CAD build for the part. Positions are in the model's coordinates, mm. Face numbers are marked on the shaded views. A direction names the side the tool comes from. Round coordinates to 2 decimals unless told otherwise and drop trailing zeros. Write each loop counter-clockwise with the first axis right and the second up, starting at its lowest first coordinate (ties: lowest second). Pieces come first, ordered by that corner, then holes. Notation, with made-up numbers: (-4.75, 9) -> (23.25, 9) arc R5 cw to (23.25, 17) -> close; hole circle Ø4 at (78, 28.5). An arc over 180 degrees is marked (long way). Put each result on its own line as item: value. Start each with the question number.
1. 3-axis set-ups, long thin cutter, end or side, ignore diameter. For the marked faces 1, 2 and 3: which of +Z, -Z, +X, -X, +Y, -Y reach the whole face in a straight line?
2. Drill centre lines: line 1 (X direction, y = 13, z = 1); line 2 (Z direction, x = 17, y = 2.5); line 3 (Z direction, x = 10.5, y = 27). Where is each one in solid material? Low to high. Write a range as from..to.
3. Saw through at A-A on y = 10. List the corners of the cut face in (x, z).
4. Saw through at D-D on x = 125. List the corners of the cut face in (y, z).
5. Saw through at C-C on z = 12.5. List the corners of the cut face in (x, y), and give its area (3 significant figures).
6. Flat gauge pins, fed straight in: P1, Ø10, axis at x = 80, z = 8, coming from the -Y side; P2, Ø4.5, axis at y = 73, z = 3, coming from the +X side; P3, Ø1.9, axis at x = -3, y = 0.5, coming from the +Z side. Where does each tip first touch, or does it go through?
7. Saw through at B-B on x = -3. List the corners of the cut face in (y, z), and give its area (3 significant figures).
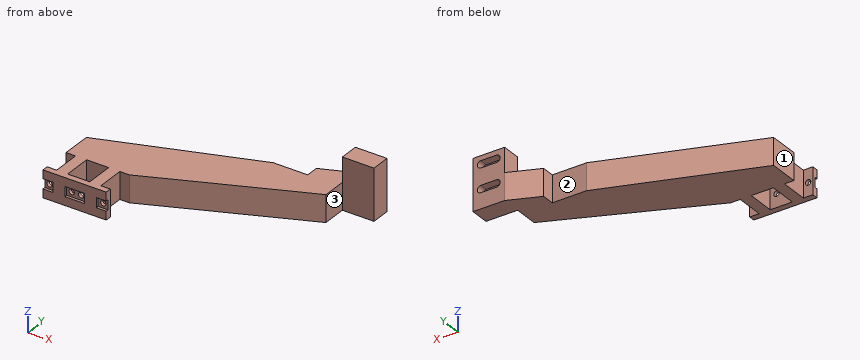
from build123d import *
from build123d.topology import SkipClean

# Parameters (mm, degrees)
EXTRUDE_1_DEPTH          = 8.5
SKETCH_2_W               = 6.2
SKETCH_2_H               = 6.2
CUT_EXTRUDE_1_DEPTH      = 1.7
SKETCH_3_W               = 6
SKETCH_3_H               = 17.5
SKETCH_3_W_2             = 14
CUT_EXTRUDE_2_DEPTH      = 164.966459985
HOLE_WIZARD_M3_1_D       = 3.4
HOLE_WIZARD_M3_1_DEPTH   = 5
HOLE_WIZARD_M3_1_TIP     = 1.021463052
SKETCH_6_W               = 20
SKETCH_6_H               = 12
EXTRUDE_2_DEPTH          = 15.4
HOLE_START               = 85
HOLE_WIZARD_M4_1_DEPTH   = 5
HOLE_START_2             = 121
HOLE_WIZARD_M4_1_2_DEPTH = 10


with BuildPart() as part:
    # 스케치1 → 보스-돌출1 (new, symmetric)
    with BuildSketch(Plane.XY):
        Polygon((20, 0), (-20, 0), (-20, 40), (75, 74), (96.8, 74), (96.8, 82), (116, 90), (136, 90), (136, 78), (116, 78), (116, 62.8), (20, 21.3), align=None)
    extrude(amount=EXTRUDE_1_DEPTH, both=True)

    # 스케치2 → 컷-돌출1 (cut)
    with BuildSketch(Plane(origin=(0, 0, 0), x_dir=(-1, 0, 0), z_dir=(0, -1, 0))):
        with Locations((-3.1, 0)):
            Rectangle(SKETCH_2_W, SKETCH_2_H)
        with Locations((-16.9, 0)):
            Rectangle(SKETCH_2_W, SKETCH_2_H)
    cut_extrude_1 = extrude(amount=-CUT_EXTRUDE_1_DEPTH, mode=Mode.SUBTRACT)

    # 대칭 복사1: 컷-돌출1 across plane
    add(cut_extrude_1.mirror(Plane(origin=(0, 0, 0), x_dir=(0, 0, 1), z_dir=(1, 0, 0))), mode=Mode.SUBTRACT)

    # 스케치3 → 컷-돌출2 (cut, through all)
    with BuildSketch(Plane(origin=(0, 0, -8.5), x_dir=(-1, 0, 0), z_dir=(0, 0, -1))):
        with Locations((-17, 12.55)):
            Rectangle(SKETCH_3_W, SKETCH_3_H)
        with Locations((0, 12.55)):
            Rectangle(SKETCH_3_W_2, SKETCH_3_H)
        with Locations((17, 12.55)):
            Rectangle(SKETCH_3_W, SKETCH_3_H)
    extrude(amount=-CUT_EXTRUDE_2_DEPTH, mode=Mode.SUBTRACT)

    # M3 여유 구멍1
    with Locations(Plane(origin=(0, 1.7, 0), x_dir=(-1, 0, 0), z_dir=(0, -1, 0))):
        with Locations((17, 0), (3, 0), (-3, 0), (-17, 0)):
            Hole(HOLE_WIZARD_M3_1_D / 2, depth=HOLE_WIZARD_M3_1_DEPTH)
            with Locations((0, 0, -(HOLE_WIZARD_M3_1_DEPTH + HOLE_WIZARD_M3_1_TIP / 2))):  # 118° drill point
                Cone(0, HOLE_WIZARD_M3_1_D / 2, HOLE_WIZARD_M3_1_TIP, mode=Mode.SUBTRACT)

    # 스케치6 → 보스-돌출2 (add)
    with BuildSketch(Plane.XY.offset(8.5)):
        with Locations((126, 84)):
            Rectangle(SKETCH_6_W, SKETCH_6_H)
    extrude(amount=EXTRUDE_2_DEPTH)

    # M4 여유 홈1: read off the stored shape, not the designer's step
    # M4 여유 홈1 outline → M4 여유 홈1 (cut)
    with BuildSketch(Plane(origin=(0, 0, 0), x_dir=(1, 0, 0), z_dir=(0, 1, 0)).offset(HOLE_START)):
        with BuildLine():
            Line((121, -5.85), (131, -5.85))
            ThreePointArc((131, -5.85), (133.25, -3.6), (131, -1.35))
            Line((131, -1.35), (121, -1.35))
            ThreePointArc((121, -1.35), (118.75, -3.6), (121, -5.85))
        make_face()
        with BuildLine():
            Line((121, -20.85), (131, -20.85))
            ThreePointArc((131, -20.85), (133.25, -18.6), (131, -16.35))
            Line((131, -16.35), (121, -16.35))
            ThreePointArc((121, -16.35), (118.75, -18.6), (121, -20.85))
        make_face()
    extrude(amount=HOLE_WIZARD_M4_1_DEPTH, mode=Mode.SUBTRACT)

    # Hole Wizard M4 _ _1 2 outline → Hole Wizard M4 _ _1 2 (cut)
    with BuildSketch(Plane.YZ.offset(HOLE_START_2)):
        Polygon((85, 5.85), (83.648063607, 3.6), (85, 1.35), align=None)
        Polygon((85, 20.85), (83.648063607, 18.6), (85, 16.35), align=None)
    extrude(amount=HOLE_WIZARD_M4_1_2_DEPTH, mode=Mode.SUBTRACT)

    # Hole Wizard M4 _ _1 3 outline → Hole Wizard M4 _ _1 3 (revolve, cut)
    with SkipClean():  # the faces are left unmerged after this step: merging them gives an invalid solid
        with BuildSketch(Plane(origin=(131, 0, 3.6), x_dir=(1, 0, 0), z_dir=(0, 0, 1))):
            Polygon((0, 85), (0, 83.648063607), (2.25, 85), align=None)
        revolve(axis=Axis((131, 0, 3.6), (0, 1, 0)), mode=Mode.SUBTRACT)

    # Hole Wizard M4 _ _1 4 outline → Hole Wizard M4 _ _1 4 (revolve, cut)
    with SkipClean():  # the faces are left unmerged after this step: merging them gives an invalid solid
        with BuildSketch(Plane(origin=(121, 0, 3.6), x_dir=(1, 0, 0), z_dir=(0, 0, 1))):
            Polygon((0, 85), (0, 83.648063607), (2.25, 85), align=None)
        revolve(axis=Axis((121, 0, 3.6), (0, 1, 0)), mode=Mode.SUBTRACT)

    # Hole Wizard M4 _ _1 5 outline → Hole Wizard M4 _ _1 5 (revolve, cut)
    with SkipClean():  # the faces are left unmerged after this step: merging them gives an invalid solid
        with BuildSketch(Plane(origin=(131, 0, 18.6), x_dir=(1, 0, 0), z_dir=(0, 0, 1))):
            Polygon((0, 85), (0, 83.648063607), (2.25, 85), align=None)
        revolve(axis=Axis((131, 0, 18.6), (0, 1, 0)), mode=Mode.SUBTRACT)

    # Hole Wizard M4 _ _1 6 outline → Hole Wizard M4 _ _1 6 (revolve, cut)
    with SkipClean():  # the faces are left unmerged after this step: merging them gives an invalid solid
        with BuildSketch(Plane(origin=(121, 0, 18.6), x_dir=(1, 0, 0), z_dir=(0, 0, 1))):
            Polygon((0, 85), (0, 83.648063607), (2.25, 85), align=None)
        revolve(axis=Axis((121, 0, 18.6), (0, 1, 0)), mode=Mode.SUBTRACT)


solid = part.part
Return value:
1. face 1: +Z, -Z, -X, +Y, -Y
1. face 2: +Z, -Z, -X, +Y
1. face 3: +Z, -Z, +X, -Y
2. line 1: x = -14..-7, 7..14
2. line 2: z = -8.5..-1.7, 1.7..8.5
2. line 3: z = -8.5..8.5
3. outline: (-14, -8.5) -> (-7, -8.5) -> (-7, 8.5) -> (-14, 8.5) -> close; (7, -8.5) -> (14, -8.5) -> (14, 8.5) -> (7, 8.5) -> close
4. outline: (78, -8.5) -> (90, -8.5) -> (90, 1.35) -> (85, 1.35) -> (83.65, 3.6) -> (85, 5.85) -> (90, 5.85) -> (90, 16.35) -> (85, 16.35) -> (83.65, 18.6) -> (85, 20.85) -> (90, 20.85) -> (90, 23.9) -> (78, 23.9) -> close
5. outline: (116, 78) -> (136, 78) -> (136, 90) -> (116, 90) -> close
5. area: 240 mm^2
6. P1: stops at y = 45.08
6. P2: stops at x = 116
6. P3: stops at z = 8.5
7. outline: (0, -8.5) -> (3.8, -8.5) -> (3.8, -1.7) -> (1.7, -1.7) -> (1.7, -3.1) -> (0, -3.1) -> close; (0, 3.1) -> (1.7, 3.1) -> (1.7, 1.7) -> (3.8, 1.7) -> (3.8, 8.5) -> (0, 8.5) -> close; (21.3, -8.5) -> (46.08, -8.5) -> (46.08, 8.5) -> (21.3, 8.5) -> close
7. area: 468 mm^2
